```python
from build123d import *

# Parameters (mm, degrees)
F1_DEPTH = 15
F2_R     = 10
F4_DEPTH = 10
F6_DEPTH = 10


with BuildPart() as f1:
    # F0 (on Front) → F1 (new body, symmetric)
    with BuildSketch(Plane.XZ):
        with BuildLine():
            Line((-50, 10), (-50, 0))
            Line((-50, 0), (-25, 0))
            Line((-25, 0), (-25, -5))
            Line((-25, -5), (-20, -5))
            Line((-20, -5), (-20, 0))
            ThreePointArc((-20, 0), (0, 20), (20, 0))
            Line((20, 0), (20, -5))
            Line((20, -5), (25, -5))
            Line((25, -5), (25, 0))
            Line((25, 0), (50, 0))
            Line((50, 0), (50, 10))
            Line((50, 10), (28.284271, 10))
            ThreePointArc((28.284271, 10), (0, 30), (-28.284271, 10))
            Line((-28.284271, 10), (-50, 10))
        make_face()
    extrude(amount=F1_DEPTH, both=True)

    # F2
    f2_edges = [f1.edges().sort_by_distance(p)[0] for p in [
        (-50, -15, 5),
        (50, -15, 5),
        (50, 15, 5),
        (-50, 15, 5),
    ]]
    fillet(f2_edges, radius=F2_R)

    # F3 (on face) → F4 (cut, through all)
    with BuildSketch(Plane.XY.offset(10)):
        with BuildLine():
            Line((-40, 5), (-50, 5))
            Line((-50, 5), (-50, -5))
            Line((-50, -5), (-40, -5))
            ThreePointArc((-40, -5), (-35, 0), (-40, 5))
        make_face()
    extrude(amount=-F4_DEPTH, mode=Mode.SUBTRACT)

    # F5 (on face) → F6 (cut, through all)
    with BuildSketch(Plane.XY.offset(10)):
        with BuildLine():
            Line((50, -5), (50, 5))
            Line((50, 5), (40, 5))
            ThreePointArc((40, 5), (35, 0), (40, -5))
            Line((40, -5), (50, -5))
        make_face()
    extrude(amount=-F6_DEPTH, mode=Mode.SUBTRACT)


solid = f1.part
```
For this review, take the finished solid that the model builds, in its own axes (mm). A direction names the side the tool comes from. Coordinates: 2 decimals unless noted, no trailing zeros. Loops run counter-clockwise (first coordinate to the right, second up) from the corner with the lowest first, then second, coordinate; pieces in that order, holes last. Notation, with made-up numbers: (-8.5, 13.25) -> (7.5, 13.25) arc R26 ccw to (7.5, 33.25) -> close; hole circle Ø9 at (80, 5.25). An arc over 180 degrees is marked (long way). Return JSON: item names as keys, results as strings. Group by question number.
(1) For pin 1 Ø4 at (y, z) = (-8.5, 18) entering from -X; pin 2 Ø1.5 at (y, z) = (0.5, 7.5) entering from -X; pin 3 Ø5 at (x, z) = (45, 6.5) entering from -Y; pin 4 Ø11 at (x, z) = (-45, 5) entering from -Y, all flat-tipped, find the tip position at first contact; note any pin that passes through.
(2) Consider section D-D, the plane x = 24. Give the boundary of the cut face in (y, z), plus the area to 3 significant figures.
(3) Mouldability with a two-part tool opening along Y and no side actions: class faces 1 (the flat face through (34, 0, 10)), 2 (the cylindrical face through (47.15, 11.99, 5.07)), 3 (the flat face through (-45, -5, 5)) as pulls with the +Y half, pulls with the -Y half, needs draft (parallel to the pull), parting line crosses it, or undercut.
(4) To check wall thickness, follow L1, parallel to X at y = 10.5, z = -1; L2, parallel to Z at x = 31, y = 3.5; L3, parallel to Y at x = -44, z = 6. State the ranges of each line that lie inside material, in increasing order.
(5) Consider section B-B, the plane x = -44. Give the boundary of the cut face in (y, z), plus the area to 3 significant figures.
(6) Consider section A-A, the plane z = -2. Give the boundary of the cut face in (x, y), plus the area to 3 significant figures.
(7) Consider section C-C, the plane y = 3. Give the boundary of the cut face in (x, z), plus the area to 3 significant figures.
(8) Tool access review of faces 4 (the flat face through (25, 0, -3)), 5 (the flat face through (-20, 0, -3)), 6 (the flat face through (-45, 5, 5)): name each direction out of +Z, -Z, +X, -X, +Y, -Y from which nothing blocks a thin tool from reaching the whole face with its end or side.
Results below:
{
 "1": {"pin 1": "stops at x = -25.38", "pin 2": "stops at x = -35.16", "pin 3": "stops at y = -14.68", "pin 4": "stops at y = -15"},
 "2": {"outline": "(-15, -5) -> (15, -5) -> (15, 18) -> (-15, 18) -> close", "area": "690 mm2"},
 "3": {"face 1": "needs draft", "face 2": "pulls with the +Y half", "face 3": "undercut"},
 "4": {"L1": "x = -25 to -20, 20 to 25", "L2": "z = 0 to 10", "L3": "y = -14.17 to -5, 5 to 14.17"},
 "5": {"outline": "(-14.17, 0) -> (-5, 0) -> (-5, 10) -> (-14.17, 10) -> close; (5, 0) -> (14.17, 0) -> (14.17, 10) -> (5, 10) -> close", "area": "183 mm2"},
 "6": {"outline": "(-25, -15) -> (-20, -15) -> (-20, 15) -> (-25, 15) -> close; (20, -15) -> (25, -15) -> (25, 15) -> (20, 15) -> close", "area": "300 mm2"},
 "7": {"outline": "(-36, 0) -> (-25, 0) -> (-25, -5) -> (-20, -5) -> (-20, 0) arc R20 cw to (20, 0) -> (20, -5) -> (25, -5) -> (25, 0) -> (36, 0) -> (36, 10) -> (28.28, 10) arc R30 ccw to (-28.28, 10) -> (-36, 10) -> close", "area": "967 mm2"},
 "8": {"face 4": "-Z, +X, +Y, -Y", "face 5": "-Z, +Y, -Y", "face 6": "+Z, -Z, -X"}
}
